Part model, mm, in its own coordinate system. A direction names the side the tool comes from. Coordinates: 2 decimals unless noted, no trailing zeros. Write each loop counter-clockwise with the first axis right and the second up, starting at its lowest first coordinate (ties: lowest second). Pieces come first, ordered by that corner, then holes. Notation, with made-up numbers: M 38,34.5 L 51,34.5 A24 cw 51,59.5 Z; hole C 39.25,-17.75 d1. An arc over 180 degrees is marked long. Use a Markdown table: item, result. Add a question column.
Q1. Slice it at A-A on z = 0. Write the cut outline in (x, y).
Q2. Tool access for faces 5 (the flat face through (10, -27.6, 11)), 6 (the cylindrical face through (-7.47, -4.93, -15.62)), 7 (the flat face through (12, -10, -4)): list every direction of +Z, -Z, +X, -X, +Y, -Y with a clear straight run to the whole face (end or side of a thin tool).
Q3. Wall check: L1, parallel to Z at x = 10, y = -19; L2, parallel to Z at x = -0.5, y = -22.5; L3, parallel to X at y = -8.5, z = 10.5. Give the ranges that are in metal, low to high. Write a range as from..to.
Q4. Slice it at B-B on y = -20. Write the cut outline in (x, z).
Q5. Mould opens along X. For faces 1 (the flat face through (11, -36, -11)), 2 (the cylindrical face through (-18.468, -26.789, -11.257)), 3 (the cylindrical face through (-7.57, -31.495, -17.035)), 4 (the cylindrical face through (-5.615, -17.755, -25.284)) say: released by +X, released by -X, zero draft, split by the parting line, or undercut.
Q6. Pin check, flat tips, straight feed: pin 1 Ø10 at (x, y) = (-4.5, -6) entering from +Z; pin 2 Ø1 at (x, y) = (-18, -12.5) entering from -Z; pin 3 Ø1 at (y, z) = (-7.5, 3.5) entering from +X; pin 4 Ø21 at (x, z) = (-3.79, 0) entering from -Y. Stop position of each tip, or through.
from build123d import *

# Parameters (mm, degrees)
F0_R     = 25.9
F0_R_2   = 16
F1_DEPTH = 10
F3_R     = 25.9
F3_R_2   = 17.45
F4_DEPTH = 16
F5_R     = 25.9
F5_R_2   = 18.5
F6_DEPTH = 1.6
F7_R     = 25.9
F7_R_2   = 18.5
F7_R_3   = 17.45
F8_DEPTH = 8.4
F9_SIZE  = 0.5
F10_SIZE = 0.5
F11_SIZE = 0.5


# Not quite as in the source:
# - a feature names something its author has since deleted; it is built from what else it names


with BuildPart() as f1:
    # F0 (on Front) → F1 (new body)
    with BuildSketch(Plane.XZ):
        Circle(F0_R)
        with Locations((-4, 0)):
            Circle(F0_R_2, mode=Mode.SUBTRACT)
    extrude(amount=F1_DEPTH)

    # F3 (on face) → F4 (join)
    with BuildSketch(Plane.XZ.offset(10)):
        Circle(F3_R)
        with Locations((-3.7866821816, 0)):
            Circle(F3_R_2, mode=Mode.SUBTRACT)
    extrude(amount=F4_DEPTH)

    # F5 (on face) → F6 (join)
    with BuildSketch(Plane.XZ.offset(26)):
        Circle(F5_R)
        with Locations((-3.7866821816, 0)):
            Circle(F5_R_2, mode=Mode.SUBTRACT)
    extrude(amount=F6_DEPTH)

    # F7 (on face) → F8 (join)
    with BuildSketch(Plane.XZ.offset(27.6)):
        Circle(F7_R)
        with Locations((-3.7866821816, 0)):
            Circle(F7_R_2, mode=Mode.SUBTRACT)
        with Locations((-3.7866821816, 0)):
            Circle(F7_R_2)
        with Locations((-3.7866821816, 0)):
            Circle(F7_R_3, mode=Mode.SUBTRACT)
    extrude(amount=F8_DEPTH)

    # F9
    f9_edges = [f1.edges().sort_by_distance(p)[0] for p in [
        (-25.9, 0, 0),
    ]]
    chamfer(f9_edges, length=F9_SIZE)

    # F10
    f10_edges = [f1.edges().sort_by_distance(p)[0] for p in [
        (-25.9, -36, 0),
    ]]
    chamfer(f10_edges, length=F10_SIZE)

    # F11
    f11_edges = [f1.edges().sort_by_distance(p)[0] for p in [
        (-21.236682, -36, 0),
    ]]
    chamfer(f11_edges, length=F11_SIZE)


solid = f1.part
Recorded:
| question | item | result |
|---|---|---|
| 1 | outline | M -25.9,-35.5 L -25.4,-36 L -21.74,-36 L -21.24,-35.5 L -21.24,-27.6 L -22.29,-27.6 L -22.29,-26 L -21.24,-26 L -21.24,-10 L -20,-10 L -20,0 L -25.4,0 L -25.9,-0.5 Z; M 12,-10 L 13.66,-10 L 13.66,-26 L 14.71,-26 L 14.71,-27.6 L 13.66,-27.6 L 13.66,-35.5 L 14.16,-36 L 25.4,-36 L 25.9,-35.5 L 25.9,-0.5 L 25.4,0 L 12,0 Z |
| 2 | face 5 | none |
| 2 | face 6 | +Y, -Y |
| 2 | face 7 | -Y |
| 3 | L1 | -23.89..-10.7, 10.7..23.89 |
| 3 | L2 | -25.9..-17.14, 17.14..25.9 |
| 3 | L3 | -23.68..-16.07, 8.07..23.68 |
| 4 | outline | C 0,0 d51.8; hole C -3.79,0 d34.9 |
| 5 | face 1 | zero draft |
| 5 | face 2 | undercut |
| 5 | face 3 | undercut |
| 5 | face 4 | split by the parting line |
| 6 | pin 1 | z = 25.9 |
| 6 | pin 2 | z = -19.09 |
| 6 | pin 3 | x = 25.73 |
| 6 | pin 4 | through |
